```python
from build123d import *

# Parameters (mm, degrees)
BOSS_EXTRUDE1_DEPTH       = 36
SKETCH1_3_R               = 11
BOSS_EXTRUDE2_DEPTH       = 2
M3X0_5_TAPPED_HOLE1_D     = 2.5
M3X0_5_TAPPED_HOLE1_DEPTH = 5
M3X0_5_TAPPED_HOLE1_TIP   = 0.751075774
BOSS_EXTRUDE3_DEPTH       = 21
SKETCH4_W                 = 5
SKETCH4_H                 = 10
BOSS_EXTRUDE4_DEPTH       = 3
BOSS_EXTRUDE5_START       = 3
SKETCH4_3_R               = 1.25
BOSS_EXTRUDE5_DEPTH       = 2


with BuildPart() as part:
    # Sketch1 → Boss-Extrude1 (new body)
    with BuildSketch(Plane.XY):
        Polygon((-14.5, 17.5), (-17.5, 14.5), (-17.5, -14.5), (-14.5, -17.5), (14.5, -17.5), (17.5, -14.5), (17.5, 14.5), (14.5, 17.5), align=None)
    extrude(amount=-BOSS_EXTRUDE1_DEPTH)

    # Sketch1<3> → Boss-Extrude2 (add)
    with BuildSketch(Plane.XY):
        Circle(SKETCH1_3_R)
    extrude(amount=BOSS_EXTRUDE2_DEPTH)

    # M3x0.5 Tapped Hole1
    with Locations(Plane.XY):
        with Locations((13, 13), (-13, 13), (-13, -13), (13, -13)):
            Hole(M3X0_5_TAPPED_HOLE1_D / 2, depth=M3X0_5_TAPPED_HOLE1_DEPTH)
            with Locations((0, 0, -(M3X0_5_TAPPED_HOLE1_DEPTH + M3X0_5_TAPPED_HOLE1_TIP / 2))):  # 118° drill point
                Cone(0, M3X0_5_TAPPED_HOLE1_D / 2, M3X0_5_TAPPED_HOLE1_TIP, mode=Mode.SUBTRACT)

    # Sketch1<4> → Boss-Extrude3 (add)
    with BuildSketch(Plane.XY):
        with BuildLine():
            Line((-1.5, 2), (1.5, 2))
            ThreePointArc((1.5, 2), (0, -2.5), (-1.5, 2))
        make_face()
    extrude(amount=BOSS_EXTRUDE3_DEPTH)

    # Sketch4 → Boss-Extrude4 (add)
    with BuildSketch(Plane(origin=(17.5, 0, 0), x_dir=(0, 0, -1), z_dir=(1, 0, 0))):
        with Locations((33.5, 0)):
            Rectangle(SKETCH4_W, SKETCH4_H)
    extrude(amount=BOSS_EXTRUDE4_DEPTH)

    # Sketch4<3> → Boss-Extrude5 (add)
    with BuildSketch(Plane(origin=(17.5, 0, 0), x_dir=(0, 0, -1), z_dir=(1, 0, 0)).offset(BOSS_EXTRUDE5_START)):
        with Locations((33.5, 3)):
            Circle(SKETCH4_3_R)
        with Locations((33.5, 1)):
            Circle(SKETCH4_3_R)
        with Locations((33.5, -1)):
            Circle(SKETCH4_3_R)
        with Locations((33.5, -3)):
            Circle(SKETCH4_3_R)
    extrude(amount=BOSS_EXTRUDE5_DEPTH)


solid = part.part
```
Geometry: final body of the model. Coordinates: model frame, mm. A direction names the side the tool comes from. Coordinates: 2 decimals unless noted, no trailing zeros. Order: outer loops, then holes, each group sorted by start corner. A loop starts at its lowest first (then second) coordinate and runs counter-clockwise, first axis right, second up. Notation, with made-up numbers: (-38.5, -0.75) -> (1.5, -0.75) arc R24 cw to (1.5, 31.25) -> close; hole circle Ø3 at (60.25, 11). An arc over 180 degrees is marked (long way). Write each question's results on one line, items separated by ' | '. Start each with the question number.
1) Cut plane C-C, the plane x = 16. Output: boundary loops of the cut face in (y, z).
2) Cut plane A-A, the plane z = -33.5. Output: boundary loops of the cut face in (x, y), and give its area (3 significant figures).
3) Material intervals for line 1 along X through (y, z) = (-13, -3.2); line 2 along X through (y, z) = (5.5, -19), sorted ascending.
4) First-contact query: pin 1 (0.9 mm diameter, centred on x = 18.5, z = -34, fed in from -Y); pin 2 (2.5 mm diameter, centred on x = 18.5, z = -33, fed in from +Y); pin 3 (4 mm diameter, centred on x = -13, y = 13, fed in from +Z); pin 4 (5 mm diameter, centred on x = 5.5, z = 6, fed in from +Y). Flat tips, straight axial feed; report the tip coordinate or a pass-through.
5) Set-up query: faces 4 (the flat face through (0, 2, 11)), 5 (the flat face through (-17.5, 0, -18)), 6 (the cylindrical face through (13.921, -12.155, -2.535)), 7 (the flat face through (19, 0, -31)). Return all of +Z, -Z, +X, -X, +Y, -Y with unobstructed straight access to the full face (end or side cutting, diameter ignored); none if empty.
6) Cut plane D-D, the plane x = 9.5. Output: boundary loops of the cut face in (y, z).
7) Mould query, pull axis X, two halves, no side actions, for faces 1 (the cylindrical face through (13.16, 14.24, -2.54)), 2 (the cylindrical face through (0.1, -2.5, 11.4)), 3 (the flat face through (16, -16, -18)). Classes: released by +X, released by -X, zero draft, split by the parting line, or undercut.
8) Cut plane B-B, the plane y = -6. Output: boundary loops of the cut face in (x, z).
Checks:
1) outline: (-16, -36) -> (16, -36) -> (16, 0) -> (-16, 0) -> close
2) outline: (-17.5, -14.5) -> (-14.5, -17.5) -> (14.5, -17.5) -> (17.5, -14.5) -> (17.5, -5) -> (20.5, -5) -> (20.5, -4.25) -> (22.5, -4.25) -> (22.5, 4.25) -> (20.5, 4.25) -> (20.5, 5) -> (17.5, 5) -> (17.5, 14.5) -> (14.5, 17.5) -> (-14.5, 17.5) -> (-17.5, 14.5) -> close | area: 1,250 mm^2
3) line 1: -17.5 to -14.25, -11.75 to 11.75, 14.25 to 17.5 | line 2: -17.5 to 17.5
4) pin 1: y = -5 | pin 2: y = 14.75 | pin 3: z = 0 | pin 4: through
5) face 4: +Z, +X, -X, +Y | face 5: +Z, -Z, -X, +Y, -Y | face 6: +Z | face 7: +Z, +X, +Y, -Y
6) outline: (-17.5, -36) -> (17.5, -36) -> (17.5, 0) -> (5.55, 0) -> (5.55, 2) -> (-5.55, 2) -> (-5.55, 0) -> (-17.5, 0) -> close
7) face 1: undercut | face 2: split by the parting line | face 3: released by +X
8) outline: (-17.5, -36) -> (17.5, -36) -> (17.5, 0) -> (9.22, 0) -> (9.22, 2) -> (-9.22, 2) -> (-9.22, 0) -> (-17.5, 0) -> close
